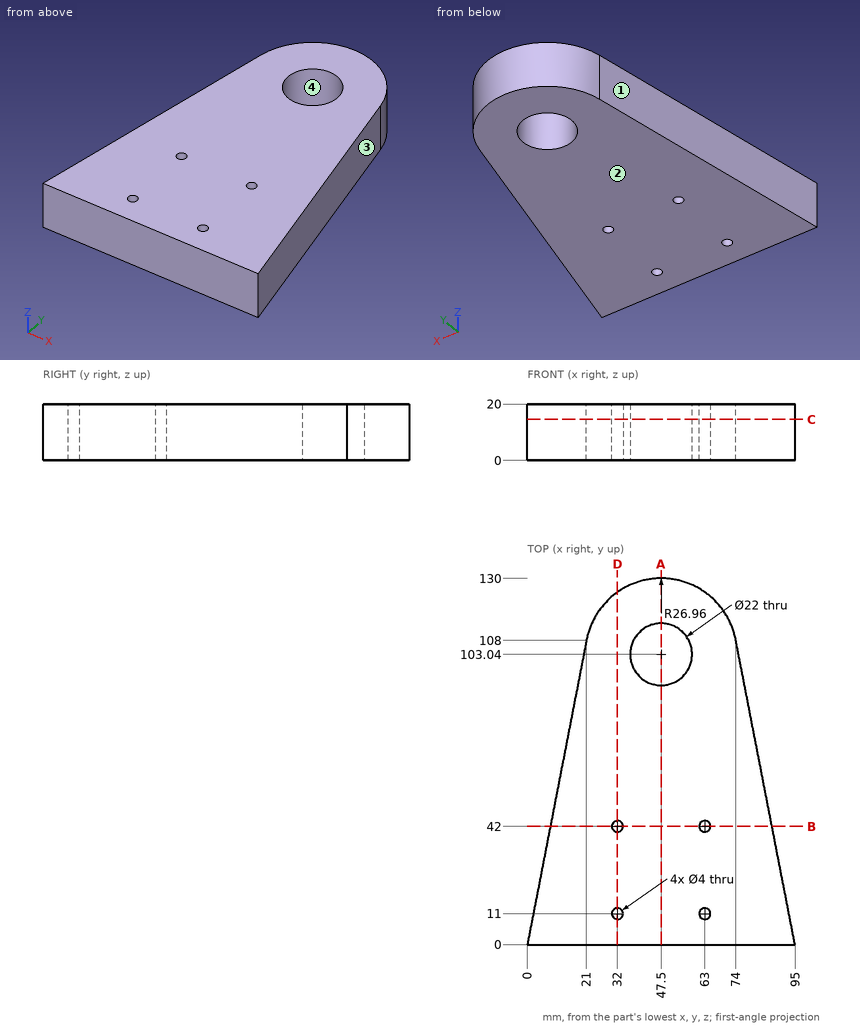
Could you check a few things on this drawing? It's one solid part, dimensions in mm from its lowest x, y, z. Coordinates: 2 decimals unless noted, no trailing zeros. Order: outer loops, then holes, each group sorted by start corner. A loop starts at its lowest first (then second) coordinate and runs counter-clockwise, first axis right, second up. Notation, with made-up numbers: M 16,16.5 L 37,16.5 A28 ccw 37,48.5 Z; hole C 48.5,35.5 d8. An arc over 180 degrees is marked long. Answer as a JSON object with one key per item and string values. Group by question number.
(1) Suppose I cut it at D-D, the plane x = 32. Please give me the cut outline in (y, z).
(2) For pin 1 (2 mm diameter, centred on y = 94.5, z = 17.5, fed in from +X); pin 2 (3 mm diameter, centred on x = 67.5, z = 15.5, fed in from -Y); pin 3 (5 mm diameter, centred on y = 66, z = 15, fed in from +X); pin 4 (2 mm diameter, centred on x = 44, z = 8, fed in from +Y), each with a flat end and sliding along its axis, tell me the tip position at first contact or that it passes through.
(3) If we mould it in two halves opening along X, with no side actions, what happens to the marked faces 1, 2, 3 and 4? For each: released by +X, released by -X, zero draft, split by the parting line, or undercut.
(4) Suppose I cut it at C-C, the plane z = 14.5. Please give me the cut outline in (x, y), then the cut area to 3 significant figures.
(5) Suppose I cut it at B-B, the plane y = 42. Please give me the cut outline in (x, z).
(6) Suppose I cut it at A-A, the plane x = 47.5. Please give me the cut outline in (y, z).
(7) I need wall thicknesses on probe 1 along Y at (x, z) = (63, 9.25); probe 2 along Y at (x, z) = (47.5, 9.75); probe 3 along Y at (x, z) = (50.5, 19.25). Which ranges of each line are inside material? Lowest first, please.
Values found:
{
 "1": {"outline": "M 0,0 L 9,0 L 9,20 L 0,20 Z; M 13,0 L 40,0 L 40,20 L 13,20 Z; M 44,0 L 125.1,0 L 125.1,20 L 44,20 Z"},
 "2": {"pin 1": "stops at x = 76.82", "pin 2": "stops at y = 0", "pin 3": "stops at x = 82.65", "pin 4": "stops at y = 129.88"},
 "3": {"face 1": "released by -X", "face 2": "zero draft", "face 3": "released by +X", "face 4": "undercut"},
 "4": {"outline": "M 0,0 L 95,0 L 74,108 A26.96 ccw 21,108 Z; hole C 32,11 d4; hole C 32,42 d4; hole C 47.5,103.04 d22; hole C 63,11 d4; hole C 63,42 d4", "area": "8,440 mm^2"},
 "5": {"outline": "M 8.17,0 L 30,0 L 30,20 L 8.17,20 Z; M 34,0 L 61,0 L 61,20 L 34,20 Z; M 65,0 L 86.83,0 L 86.83,20 L 65,20 Z"},
 "6": {"outline": "M 0,0 L 92.04,0 L 92.04,20 L 0,20 Z; M 114.04,0 L 130,0 L 130,20 L 114.04,20 Z"},
 "7": {"probe 1": "y = 0 to 9, 13 to 40, 44 to 125.1", "probe 2": "y = 0 to 92.04, 114.04 to 130", "probe 3": "y = 0 to 92.46, 113.62 to 129.83"}
}
